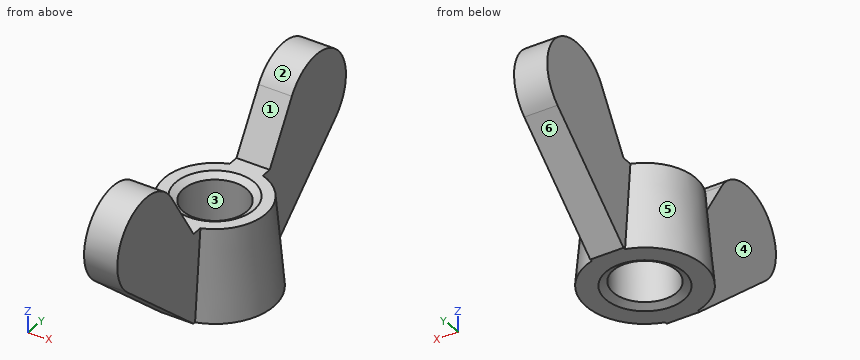
from build123d import *

# Parameters (mm, degrees)
PAD_DEPTH = 0.85


with BuildPart() as pad:
    # Sketch001 → Pad (new body, symmetric)
    with BuildSketch(Plane.YZ):
        with BuildLine():
            Line((2, 0), (2, 4.6))
            Line((2, 4.6), (3, 4.6))
            Line((3, 4.6), (4.745783, 7.412863))
            ThreePointArc((8.196676, 4.453586), (8.197219, 7.945948), (4.745783, 7.412863))
            Line((3, 0), (8.196676, 4.453586))
            Line((2, 0), (3, 0))
        make_face()
        with BuildLine():
            Line((-8.196687, 4.453578), (-3.000004, 0))
            Line((-3.000004, 0), (-2.000004, 0))
            Line((-2.000004, 0), (-2.000004, 4.6))
            Line((-2.000004, 4.6), (-3.000004, 4.6))
            Line((-3.000004, 4.6), (-4.745792, 7.41286))
            ThreePointArc((-4.745792, 7.41286), (-8.19722, 7.945929), (-8.196687, 4.453578))
        make_face()
    extrude(amount=PAD_DEPTH, both=True)


with BuildPart() as obj1:
    # Sketch → Revolution (revolve)
    with BuildSketch(Plane.YZ):
        Polygon((2, 0), (1.62, 0.219393), (1.62, 4.380607), (2, 4.6), (2.6, 4.6), (3, 0), align=None)
    revolve(axis=Axis((0, 0, 0), (0, 0, 1)))

    # Fusion: union Pad
    add(pad.part)


solid = obj1.part
The model under review builds one solid part; all positions refer to its coordinate system, in mm. Face numbers are marked on the shaded views. A direction names the side the tool comes from. Give positions to 0.01 mm unless a question says otherwise; leave off trailing zeros. Order: outer loops, then holes, each group sorted by start corner. A loop starts at its lowest first (then second) coordinate and runs counter-clockwise, first axis right, second up. Notation, with made-up numbers: M 71,31.25 L 115,31.25 A9 cw 115,44.25 Z; hole C 61.5,35 d1. An arc over 180 degrees is marked long. Answer in a Markdown table with one row per item. Add a question column.
1. Machinability: for the marked faces 1 and 2, which of the approach directions +Z, -Z, +X, -X, +Y, -Y give a long, thin tool a straight path to every point of the face, cutting with its end or side? Answer none if there is none.
2. Add section C-C on z = 1.75. State the section outline as (x, y) points.
3. Mouldability with a two-part tool opening along Y and no side actions: class the marked faces 3, 4, 5 and 6 as released by +Y, released by -Y, zero draft, split by the parting line, or undercut.
4. Add section A-A on z = 6.2. State the section outline as (x, y) points, plus the area to 3 significant figures.
5. For pin 1 Ø3 at (x, z) = (0.5, 2) entering from +Y; pin 2 Ø2.5 at (x, y) = (0, 0.5) entering from +Z; pin 3 Ø3 at (x, y) = (-1, -1) entering from +Z, all flat-tipped, find the tip position at first contact; note any pin that passes through.
6. To check wall thickness, follow line 1 along Z through (x, y) = (-0.4, 2.5); line 2 along Y through (x, z) = (0, 3.45); line 3 along Y through (x, z) = (0.25, 4.75). State the ranges of each line that lie inside material, in increasing order.
7. Add section D-D on z = 2.75. State the section outline as (x, y) points.
8. Add section B-B on y = 0. State the section outline as (x, z) points.
The answers:
| question | item | result |
|---|---|---|
| 1 | face 1 | +Z, +X, -X |
| 1 | face 2 | +X, -X |
| 2 | outline | M -0.85,-5.04 L 0.85,-5.04 L 0.85,-2.72 A2.85 ccw 0.85,2.72 L 0.85,5.04 L -0.85,5.04 L -0.85,2.72 A2.85 ccw -0.85,-2.72 Z; hole C 0,0 d3.24 |
| 3 | face 3 | undercut |
| 3 | face 4 | zero draft |
| 3 | face 5 | split by the parting line |
| 3 | face 6 | released by +Y |
| 4 | outline | M -0.85,-9 L 0.85,-9 L 0.85,-3.99 L -0.85,-3.99 Z; M -0.85,3.99 L 0.85,3.99 L 0.85,9 L -0.85,9 Z |
| 4 | area | 17.0 mm2 |
| 5 | pin 1 | y = 7.08 |
| 5 | pin 2 | z = 4.46 |
| 5 | pin 3 | z = 4.6 |
| 6 | line 1 | 0 to 4.6 |
| 6 | line 2 | -7.03 to -1.62, 1.62 to 7.03 |
| 6 | line 3 | -8.49 to -3.09, 3.09 to 8.49 |
| 7 | outline | M -0.85,-6.21 L 0.85,-6.21 L 0.85,-2.63 A2.76 ccw 0.85,2.63 L 0.85,6.21 L -0.85,6.21 L -0.85,2.63 A2.76 ccw -0.85,-2.63 Z; hole C 0,0 d3.24 |
| 8 | outline | M -3,0 L -2,0 L -1.62,0.22 L -1.62,4.38 L -2,4.6 L -2.6,4.6 Z; M 1.62,0.22 L 2,0 L 3,0 L 2.6,4.6 L 2,4.6 L 1.62,4.38 Z |
